Geometry check sheet. Reference: drawing and pictorial views, mm from the part's lowest x, y, z. A direction names the side the tool comes from. Give positions to 0.01 mm unless a question says otherwise; leave off trailing zeros. Loops run counter-clockwise (first coordinate to the right, second up) from the corner with the lowest first, then second, coordinate; pieces in that order, holes last. Notation, with made-up numbers: (34.25, 40) -> (38.25, 40) arc R33 cw to (38.25, 72) -> close; hole circle Ø8 at (-8, 87). An arc over 180 degrees is marked (long way). One line per item, written item: value. Start each with the question number.
(1) Draft check along X on the marked faces 1, 2 and 3. Enter one of: pulls with the +X half, pulls with the -X half, needs draft (parallel to the pull), parting line crosses it, or undercut.
(2) Sectioned sample at A-A, the plane x = 51. Record the cut outline in (y, z).
(3) Scan lines: line 1 along Y through (x, z) = (51, 1.05); line 2 along X through (y, z) = (5, 1.45); line 3 along Y through (x, z) = (11, 1.05). Record each from-to range of solid material in increasing order. Write a range as from..to.
(4) Sectioned sample at D-D, the plane y = 15.5. Record the cut outline in (x, z).
(5) Sectioned sample at C-C, the plane z = 9. Record the cut outline in (x, y), then the cut area to 3 significant figures.
(6) Tool access check on the marked faces 4, 5, 6 and 7. Record the directions out of +Z, -Z, +X, -X, +Y, -Y that give a thin tool (end or side, any length) a straight path to the whole face; none if there is none.
(7) Gauge pin test, flat ends, axial feed: pin 1 Ø1.5 at (x, z) = (52.5, 5.5) entering from +Y; pin 2 Ø3 at (x, z) = (22, 10) entering from -Y; pin 3 Ø1.8 at (x, y) = (1.5, 23) entering from -Z. Record the tip position at first contact, or that the pin passes through.
(8) Sectioned sample at B-B, the plane y = 5. Record the cut outline in (x, z), then the cut area to 3 significant figures.
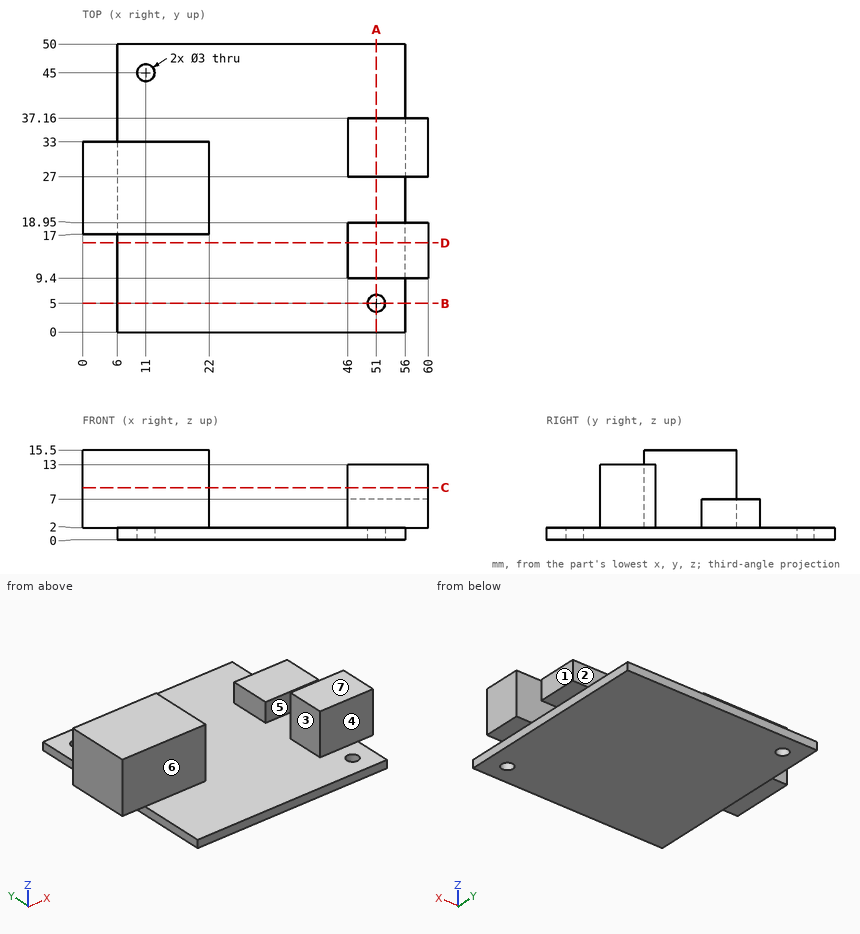
Calculated:
1. face 1: pulls with the +X half
1. face 2: needs draft
1. face 3: undercut
2. outline: (0, 0) -> (3.5, 0) -> (3.5, 2) -> (0, 2) -> close; (6.5, 0) -> (50, 0) -> (50, 2) -> (37.16, 2) -> (37.16, 7) -> (27, 7) -> (27, 2) -> (18.95, 2) -> (18.95, 13) -> (9.4, 13) -> (9.4, 2) -> (6.5, 2) -> close
3. line 1: y = 0..3.5, 6.5..50
3. line 2: x = 6..49.5, 52.5..56
3. line 3: y = 0..43.5, 46.5..50
4. outline: (6, 0) -> (56, 0) -> (56, 2) -> (60, 2) -> (60, 13) -> (46, 13) -> (46, 2) -> (6, 2) -> close
5. outline: (0, 17) -> (22, 17) -> (22, 33) -> (0, 33) -> close; (46, 9.4) -> (60, 9.4) -> (60, 18.95) -> (46, 18.95) -> close
5. area: 486 mm2
6. face 4: +Z, +X, -X, -Y
6. face 5: +Z, +X
6. face 6: +Z, -X, -Y
6. face 7: +Z, +X, +Y, -Y
7. pin 1: stops at y = 37.16
7. pin 2: stops at y = 17
7. pin 3: stops at z = 2
8. outline: (6, 0) -> (49.5, 0) -> (49.5, 2) -> (6, 2) -> close; (52.5, 0) -> (56, 0) -> (56, 2) -> (52.5, 2) -> close
8. area: 94.0 mm2
